from build123d import *

# Parameters (mm, degrees)
SKETCH_1_W          = 10.7
SKETCH_1_H          = 6
EXTRUDE_1_DEPTH     = 11.7
SKETCH_2_R          = 3.65
CUT_EXTRUDE_1_DEPTH = 18.7
CUT_EXTRUDE_2_DEPTH = 2.3
SKETCH_2_4_R        = 3.65
CUT_EXTRUDE_3_DEPTH = 15.3
CUT_EXTRUDE_4_DEPTH = 2.3
FILLET_1_R          = 2
FILLET_2_R          = 2
FILLET_3_R          = 2
FILLET_4_R          = 2
FILLET_5_R          = 5.85
FILLET_6_R          = 5.85
FILLET_7_R          = 5.85
FILLET_8_R          = 5.85
FILLET_9_R          = 5.85
FILLET_10_R         = 5.85
FILLET_11_R         = 5.85
FILLET_12_R         = 5.85
FILLET_13_R         = 2
FILLET_14_R         = 2
FILLET_15_R         = 2
FILLET_16_R         = 2
FILLET_17_R         = 2
FILLET_18_R         = 2
FILLET_19_R         = 2
FILLET_20_R         = 2
SKETCH_3_R          = 3.05
CUT_EXTRUDE_5_DEPTH = 10
FILLET_21_R         = 3
FILLET_22_R         = 3
FILLET_23_R         = 3
FILLET_24_R         = 3


with BuildPart() as part:
    # 草图1 → 凸台-拉伸1 (new body)
    with BuildSketch(Plane.XY):
        Polygon((0, 0), (0, -28), (3.5, -28), (3.5, -4), (35.5, -4), (35.5, -28), (39, -28), (39, 0), (28, 0), (28, 6), (39, 6), (39, 40.6), (35.5, 40.6), (35.5, 10), (3.5, 10), (3.5, 40.6), (0, 40.6), (0, 6), (11, 6), (11, 0), align=None)
        with Locations((19.5, 3)):
            Rectangle(SKETCH_1_W, SKETCH_1_H, mode=Mode.SUBTRACT)
    extrude(amount=EXTRUDE_1_DEPTH)

    # 草图2 → 切除-拉伸1 (cut)
    with BuildSketch(Plane.ZY):
        with Locations(Location((5.85, -22.15, 0), (0, 0, 270))):
            Circle(SKETCH_2_R)
    extrude(amount=-CUT_EXTRUDE_1_DEPTH, mode=Mode.SUBTRACT)

    # 草图2<3> → 切除-拉伸2 (cut)
    with BuildSketch(Plane.ZY):
        with BuildLine():
            ThreePointArc((8.242618438, -6.011912226), (5.85, -3.8), (3.457381562, -6.011912226))
            Line((3.457381562, -6.011912226), (2.211226126, -21.863949843))
            ThreePointArc((2.211226126, -21.863949843), (5.85, -18.5), (9.488773874, -21.863949843))
            Line((9.488773874, -21.863949843), (8.242618438, -6.011912226))
        make_face()
    extrude(amount=-CUT_EXTRUDE_2_DEPTH, mode=Mode.SUBTRACT)

    # 草图2<4> → 切除-拉伸3 (cut)
    with BuildSketch(Plane.ZY):
        with Locations(Location((5.85, 34.75, 0), (0, 0, 270))):
            Circle(SKETCH_2_4_R)
    extrude(amount=-CUT_EXTRUDE_3_DEPTH, mode=Mode.SUBTRACT)

    # 草图2<5> → 切除-拉伸4 (cut)
    with BuildSketch(Plane.ZY):
        with BuildLine():
            Line((2.211226126, 34.463949843), (3.457381562, 18.611912226))
            ThreePointArc((3.457381562, 18.611912226), (5.85, 16.4), (8.242618438, 18.611912226))
            Line((8.242618438, 18.611912226), (9.488773874, 34.463949843))
            ThreePointArc((9.488773874, 34.463949843), (5.85, 31.1), (2.211226126, 34.463949843))
        make_face()
    extrude(amount=-CUT_EXTRUDE_4_DEPTH, mode=Mode.SUBTRACT)

    # 圆角1
    fillet_1_edges = [part.edges().sort_by_distance(p)[0] for p in [
        (0, 6, 5.85),
    ]]
    fillet(fillet_1_edges, radius=FILLET_1_R)

    # 圆角2
    fillet_2_edges = [part.edges().sort_by_distance(p)[0] for p in [
        (39, 6, 5.85),
    ]]
    fillet(fillet_2_edges, radius=FILLET_2_R)

    # 圆角3
    fillet_3_edges = [part.edges().sort_by_distance(p)[0] for p in [
        (39, 0, 5.85),
    ]]
    fillet(fillet_3_edges, radius=FILLET_3_R)

    # 圆角4
    fillet_4_edges = [part.edges().sort_by_distance(p)[0] for p in [
        (0, 0, 5.85),
    ]]
    fillet(fillet_4_edges, radius=FILLET_4_R)

    # 圆角5
    fillet_5_edges = [part.edges().sort_by_distance(p)[0] for p in [
        (1.75, -28, 11.7),
    ]]
    fillet(fillet_5_edges, radius=FILLET_5_R)

    # 圆角6
    fillet_6_edges = [part.edges().sort_by_distance(p)[0] for p in [
        (1.75, -28, 0),
    ]]
    fillet(fillet_6_edges, radius=FILLET_6_R - 0.0001)  # a hair under: the kernel refuses the full size

    # 圆角7
    fillet_7_edges = [part.edges().sort_by_distance(p)[0] for p in [
        (37.25, -28, 0),
    ]]
    fillet(fillet_7_edges, radius=FILLET_7_R)

    # 圆角8
    fillet_8_edges = [part.edges().sort_by_distance(p)[0] for p in [
        (37.25, -28, 11.7),
    ]]
    fillet(fillet_8_edges, radius=FILLET_8_R - 0.0001)  # a hair under: the kernel refuses the full size

    # 圆角9
    fillet_9_edges = [part.edges().sort_by_distance(p)[0] for p in [
        (37.25, 40.6, 11.7),
    ]]
    fillet(fillet_9_edges, radius=FILLET_9_R)

    # 圆角10
    fillet_10_edges = [part.edges().sort_by_distance(p)[0] for p in [
        (37.25, 40.6, 0),
    ]]
    fillet(fillet_10_edges, radius=FILLET_10_R - 0.0001)  # a hair under: the kernel refuses the full size

    # 圆角11
    fillet_11_edges = [part.edges().sort_by_distance(p)[0] for p in [
        (1.75, 40.6, 0),
    ]]
    fillet(fillet_11_edges, radius=FILLET_11_R)

    # 圆角12
    fillet_12_edges = [part.edges().sort_by_distance(p)[0] for p in [
        (1.75, 40.6, 11.7),
    ]]
    fillet(fillet_12_edges, radius=FILLET_12_R - 0.0001)  # a hair under: the kernel refuses the full size

    # 圆角13
    fillet_13_edges = [part.edges().sort_by_distance(p)[0] for p in [
        (28, 6, 5.85),
    ]]
    fillet(fillet_13_edges, radius=FILLET_13_R)

    # 圆角14
    fillet_14_edges = [part.edges().sort_by_distance(p)[0] for p in [
        (28, 0, 5.85),
    ]]
    fillet(fillet_14_edges, radius=FILLET_14_R)

    # 圆角15
    fillet_15_edges = [part.edges().sort_by_distance(p)[0] for p in [
        (11, 6, 5.85),
    ]]
    fillet(fillet_15_edges, radius=FILLET_15_R)

    # 圆角16
    fillet_16_edges = [part.edges().sort_by_distance(p)[0] for p in [
        (11, 0, 5.85),
    ]]
    fillet(fillet_16_edges, radius=FILLET_16_R)

    # 圆角17
    fillet_17_edges = [part.edges().sort_by_distance(p)[0] for p in [
        (24.85, 6, 5.85),
    ]]
    fillet(fillet_17_edges, radius=FILLET_17_R)

    # 圆角18
    fillet_18_edges = [part.edges().sort_by_distance(p)[0] for p in [
        (24.85, 0, 5.85),
    ]]
    fillet(fillet_18_edges, radius=FILLET_18_R)

    # 圆角19
    fillet_19_edges = [part.edges().sort_by_distance(p)[0] for p in [
        (14.15, 6, 5.85),
    ]]
    fillet(fillet_19_edges, radius=FILLET_19_R)

    # 圆角20
    fillet_20_edges = [part.edges().sort_by_distance(p)[0] for p in [
        (14.15, 0, 5.85),
    ]]
    fillet(fillet_20_edges, radius=FILLET_20_R)

    # 草图3 → 切除-拉伸5 (cut)
    with BuildSketch(Plane(origin=(39, 0, 0), x_dir=(0, 0, -1), z_dir=(1, 0, 0))):
        with Locations((-5.85, 34.75)):
            Circle(SKETCH_3_R)
        with Locations((-5.85, -22.15)):
            Circle(SKETCH_3_R)
    extrude(amount=-CUT_EXTRUDE_5_DEPTH, mode=Mode.SUBTRACT)

    # 圆角21
    fillet_21_edges = [part.edges().sort_by_distance(p)[0] for p in [
        (3.5, -4, 5.85),
    ]]
    fillet(fillet_21_edges, radius=FILLET_21_R)

    # 圆角22
    fillet_22_edges = [part.edges().sort_by_distance(p)[0] for p in [
        (35.5, -4, 5.85),
    ]]
    fillet(fillet_22_edges, radius=FILLET_22_R)

    # 圆角23
    fillet_23_edges = [part.edges().sort_by_distance(p)[0] for p in [
        (35.5, 10, 5.85),
    ]]
    fillet(fillet_23_edges, radius=FILLET_23_R)

    # 圆角24
    fillet_24_edges = [part.edges().sort_by_distance(p)[0] for p in [
        (3.5, 10, 5.85),
    ]]
    fillet(fillet_24_edges, radius=FILLET_24_R)


solid = part.part
Here's how the part is built. I have some questions about the finished solid (model axes, mm). A direction names the side the tool comes from. Round coordinates to 2 decimals unless told otherwise and drop trailing zeros. Write each loop counter-clockwise with the first axis right and the second up, starting at its lowest first coordinate (ties: lowest second). Pieces come first, ordered by that corner, then holes.
1. I need wall thicknesses on L1, parallel to Y at x = 2.6, z = 5.85; L2, parallel to Y at x = 36.55, z = 5.85; L3, parallel to X at y = 27, z = 9. Which ranges of each line are inside material? Lowest first, please.
2. Suppose I cut it at C-C (z = 4.75). State how many separate pieces and enclosed holes the cut face has, and give its area (3 significant figures).
3. Suppose I cut it at B-B (y = 21). List the corners of the cut face in (x, z) for me, and give its area (3 significant figures).
4. Will these pins go through, and if not, where does the flat tip stop? pin 1 Ø3 at (x, z) = (9.5, 9) entering from +Y; pin 2 Ø4 at (x, y) = (20.5, 11.5) entering from +Z; pin 3 Ø2 at (y, z) = (23.5, 5) entering from -X; pin 4 Ø2 at (y, z) = (2.5, 3.5) entering from -X.
5. For faces 1 (the cylindrical face through (10.43, 0.6, 5.93)), 2 (the flat face through (1.134, -13.827, 2.843)), 3 (the flat face through (19, -4, 6)), which set-ups out of +Z, -Z, +X, -X, +Y, -Y let a thin tool reach every point of the face, with its end or its side?
6. If we mould it in two halves opening along X, with no side actions, what happens to faces 4 (the flat face through (11, 3, 6)), 5 (the cylindrical face through (38.4, -0.57, 5.93)), 6 (the flat face through (20, 10, 6))? For each: released by +X, released by -X, zero draft, split by the parting line, or undercut.
7. Suppose I cut it at D-D (y = -9). List the corners of the cut face in (x, z) for me.
8. Suppose I cut it at A-A (x = 31.5). List the corners of the cut face in (y, z) for me.
Answer sheet:
1. L1: y = -28 to -25.8, -18.5 to 0, 6 to 31.1, 38.4 to 40.6
1. L2: y = -28 to -25.2, -19.1 to 0, 6 to 31.7, 37.8 to 40.6
1. L3: x = 0 to 3.5, 35.5 to 39
2. separate pieces: 5
2. enclosed holes: 1
2. area: 586 mm2
3. outline: (0, 0) - (3.5, 0) - (3.5, 11.7) - (0, 11.7) - (0, 8.43) - (2.3, 8.43) - (2.3, 3.27) - (0, 3.27) - close; (35.5, 0) - (39, 0) - (39, 11.7) - (35.5, 11.7) - close
3. area: 70.0 mm2
4. pin 1: stops at y = 10
4. pin 2: stops at z = 11.7
4. pin 3: stops at x = 2.3
4. pin 4: stops at x = 10.94
5. face 1: +Z, -Z, -X
5. face 2: -X
5. face 3: +Z, -Z, -Y
6. face 4: released by -X
6. face 5: released by +X
6. face 6: undercut
7. outline: (0, 0) - (3.5, 0) - (3.5, 11.7) - (0, 11.7) - (0, 8.48) - (2.3, 8.48) - (2.3, 3.22) - (0, 3.22) - close; (35.5, 0) - (39, 0) - (39, 11.7) - (35.5, 11.7) - close
8. outline: (-4, 0) - (0, 0) - (0, 11.7) - (-4, 11.7) - close; (6, 0) - (10, 0) - (10, 11.7) - (6, 11.7) - close
